from build123d import *

# Parameters (mm, degrees)
SKETCH1_R           = 23
SKETCH1_R_2         = 3.7
BOSS_EXTRUDE1_DEPTH = 10
HOLE1_D             = 3.2


with BuildPart() as part:
    # Sketch1 → Boss-Extrude1 (new body)
    with BuildSketch(Plane.XY):
        Circle(SKETCH1_R)
        Circle(SKETCH1_R_2, mode=Mode.SUBTRACT)
    extrude(amount=BOSS_EXTRUDE1_DEPTH)

    # Hole1 (through all)
    with Locations(Plane(origin=(0, 8.45, 0), x_dir=(-1, 0, 0), z_dir=(0, 0, -1))):
        with Locations((0, 0), (-7.317914662, -12.675), (7.317914662, -12.675)):
            Hole(HOLE1_D / 2)


solid = part.part
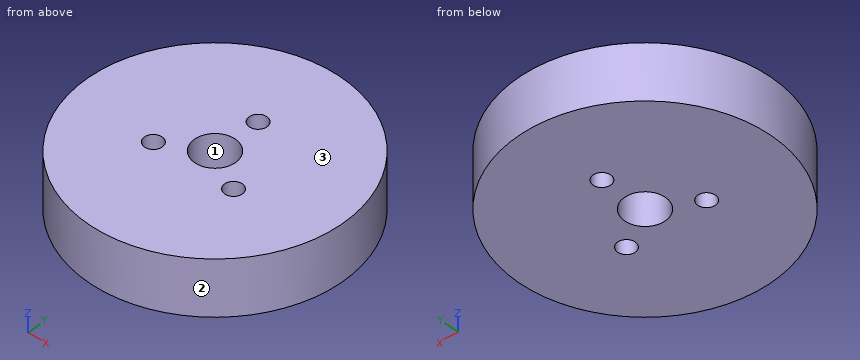
Part model, mm, in its own coordinate system. Face numbers are marked on the shaded views. Coordinates: 2 decimals unless noted, no trailing zeros. Order: outer loops, then holes, each group sorted by start corner. A loop starts at its lowest first (then second) coordinate and runs counter-clockwise, first axis right, second up. Notation, with made-up numbers: (18, 17.25) - (41, 17.25) arc R11 ccw to (41, 29.25) - close; hole circle Ø5 at (52.25, -15). An arc over 180 degrees is marked (long way). Use CSV: the item, a comma, the result in double quotes.
Item 1: Saw through at A-A on y = 0. Give the cut face in (x, z), and give its area (3 significant figures).
Solved:
outline,"(-23, 0) - (-3.7, 0) - (-3.7, 10) - (-23, 10) - close; (3.7, 0) - (23, 0) - (23, 10) - (3.7, 10) - close"
area,"386 mm²"
Item 2: Saw through at B-B on x = 0. Give the cut face in (y, z), and give its area (3 significant figures).
Solved:
outline,"(-23, 0) - (-3.7, 0) - (-3.7, 10) - (-23, 10) - close; (3.7, 0) - (6.85, 0) - (6.85, 10) - (3.7, 10) - close; (10.05, 0) - (23, 0) - (23, 10) - (10.05, 10) - close"
area,"354 mm²"
Item 3: Mould opens along X. For the marked faces 1, 2 and 3 say: +X half, -X half, draft (parallel to the pull), parting line (faces both ways), or undercut.
Solved:
face 1,"undercut"
face 2,"parting line"
face 3,"draft"
Item 4: Probe probe 1 along Y at (x, z) = (0, 6.25); probe 2 along X at (y, z) = (1.5, 4.5); probe 3 along X at (y, z) = (-19.5, 1.75). List the from-to ranges inside material, lowest first.
Solved:
probe 1,"y = -23 to -3.7, 3.7 to 6.85, 10.05 to 23"
probe 2,"x = -22.95 to -3.38, 3.38 to 22.95"
probe 3,"x = -12.2 to 12.2"
Item 5: Saw through at C-C on z = 7.5. Give the cut face in (x, y) (3 decimals), and give its area (3 significant figures).
Solved:
outline,"circle Ø46 at (0, 0); hole circle Ø3.2 at (-7.318, -4.225); hole circle Ø7.4 at (0, 0); hole circle Ø3.2 at (0, 8.45); hole circle Ø3.2 at (7.318, -4.225)"
area,"1,590 mm²"
Item 6: Drop flat-ended pins along their axis: P1, Ø4, axis at x = -3, y = -0.5, coming from the -Z side; P2, Ø2, axis at x = 6.5, z = 1.5, coming from the +Y side; P3, Ø5, axis at x = 1.5, z = 2.5, coming from the -Y side; P4, Ø3, axis at y = -9.5, z = 2, coming from the -X side. Give the stop position or say it passes through.
Solved:
P1,"stops at z = 0"
P2,"stops at y = 22.33"
P3,"stops at y = -23"
P4,"stops at x = -21.56"
Item 7: Saw through at D-D on y = 8.45. Give the cut face in (x, z), and give its area (3 significant figures).
Solved:
outline,"(-21.39, 0) - (-1.6, 0) - (-1.6, 10) - (-21.39, 10) - close; (1.6, 0) - (21.39, 0) - (21.39, 10) - (1.6, 10) - close"
area,"396 mm²"
